Geometry check sheet. Reference: the model listing, model coordinates, mm. Face numbers are marked on the shaded views. A direction names the side the tool comes from. Give positions to 0.01 mm unless a question says otherwise; leave off trailing zeros. Loops run counter-clockwise (first coordinate to the right, second up) from the corner with the lowest first, then second, coordinate; pieces in that order, holes last. Notation, with made-up numbers: (66, 22.25) -> (103, 22.25) arc R25 ccw to (103, 58.25) -> close; hole circle Ø1 at (83.25, -34.75). An arc over 180 degrees is marked (long way). Answer in a Markdown table with one row per item. Add a question column.
Autodesk Inventor part; units mm, degrees
ref_plane "YZ Plane" through (0, 0, 0) normal (1, 0, 0) x (0, 1, 0)
ref_plane "XZ Plane" through (0, 0, 0) normal (0, 1, 0) x (-1, 0, 0)
ref_plane "XY Plane" through (0, 0, 0) normal (0, 0, 1) x (1, 0, 0)
sketch "Sketch1" plane through (0, 0, 0) normal (0, 1, 0) x (-1, 0, 0)
  line L0 (0, 0) -> (203.2, 0)
  line L1 (203.2, 0) -> (203.2, 25.4)
  line L2 (203.2, 25.4) -> (0, 25.4) construction
  line L3 (0, 25.4) -> (0, 0)
  line L4 (11.45, 12.7) -> (77.45, 12.7) construction
  circle A0 centre (11.45, 12.7) radius 3.302
  circle A1 centre (77.45, 12.7) radius 3.302
  line L5 (44.45, 25.4) -> (44.45, 0) construction
  circle A2 centre (127, 12.7) radius 3.302
  circle A3 centre (177.8, 12.7) radius 3.302
  line L6 (127, 12.7) -> (177.8, 12.7) construction
  line L7 (152.4, 25.4) -> (152.4, 0) construction
  line L8 (0, 25.4) -> (0, 101.6)
  line L9 (0, 101.6) -> (203.2, 101.6)
  line L10 (203.2, 101.6) -> (203.2, 25.4)
  point P0 (44.45, 12.7)
  point P1 (152.4, 12.7)
  dimension "d0" = 66
  dimension "d1" = 6.604
  dimension "d2" = 6.604
  dimension "d3" = 25.4
  dimension "d4" = 44.45
  dimension "d6" = 50.8
  dimension "d7" = 50.8
  dimension "d8" = 76.2
  dimension "d9" = 203.2
extrude "Plate1" add sketch "Sketch1" along normal blind 3.175
sketch "Sketch2" plane through (-203.2, 3.175, 98.425) normal (0, 0, 1) x (1, 0, 0)
  line L0 (203.2, 0) -> (0, 0)
  line L1 (0, 0) -> (0, -50.8)
  line L2 (0, -50.8) -> (203.2, -50.8)
  line L3 (203.2, -50.8) -> (203.2, 0)
edge flange "Flange1" height 50.8 angle 90 thickness 3.175 bend radius 1.27 thickness toward (0, 0, 1) relief tear relief width 3.175 relief depth 1.5875 edges at (-101.6, 0, 101.6) wall of the first edge with corners at (0, 3.175, 98.425) (-203.2, 3.175, 98.425) (-203.2, -47.625, 98.425) (0, -47.625, 98.425)
bend "Bend1"
corner "Corner1"
equation "\"d11\" = BendReliefWidth"
equation "\"d12\" = BendReliefDepth"
equation "\"d13\" = MinimumRemnant"
equation "\"d14\" = BendRadius"
equation "\"d18\" = CornerReliefSize"
equation "\"d19\" = GapSize"
equation "\"d20\" = JacobiRadiusSize"
equation "\"BendRadius\" = Thickness"
equation "\"BendReliefWidth\" = Thickness"
equation "\"BendReliefDepth\" = 0.5 * Thickness"
equation "\"CornerReliefSize\" = 4 * Thickness"
equation "\"MinimumRemnant\" = 2 * Thickness"
equation "\"TransitionRadius\" = BendRadius"
equation "\"JacobiRadiusSize\" = BendRadius"
equation "\"GapSize\" = Thickness"
equation "\"d10\" = BendRadius"
properties part number "Electrical Board Mount Part1" material "Aluminum 6061"
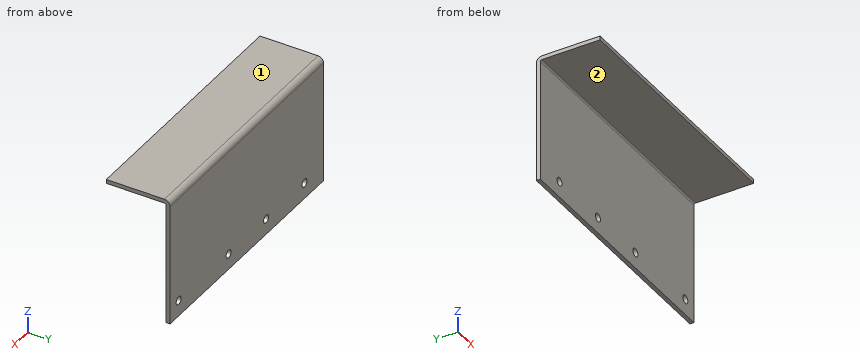
1. Sectioned sample at D-D (y = -44). Enter the section's corners in (x, z) (3 decimals).
2. Sectioned sample at B-B (x = -47). Enter the section's corners in (y, z) (3 decimals), plus the area to 3 significant figures.
3. Access from +Z, -Z, +X, -X, +Y, -Y to the whole of each face (thin tool, end or side, straight path). Record for the marked faces 1 and 2.
4. Gauge pin test, flat ends, axial feed: pin 1 Ø10.5 at (x, z) = (-127, 12.7) entering from -Y; pin 2 Ø4 at (x, y) = (-105, -13) entering from -Z (3 decimals). Record the tip position at first contact, or that the pin passes through.
5. Sectioned sample at C-C (z = 39). Enter the section's corners in (x, y) (3 decimals), plus the area to 3 significant figures.
6. Sectioned sample at A-A (x = -77.45). Enter the section's corners in (y, z) (3 decimals).
7. Material ranges on L1, parallel to Y at x = -111, z = 73 (3 decimals); L2, parallel to Z at x = -77.45, y = 0.7; L3, parallel to Z at x = -65, y = -21 (3 decimals), recorded low to high. Write a range as from..to.
Response:
| question | item | result |
|---|---|---|
| 1 | outline | (-203.2, 98.425) -> (0, 98.425) -> (0, 101.6) -> (-203.2, 101.6) -> close |
| 2 | outline | (-47.625, 98.425) -> (-1.27, 98.425) arc R1.27 cw to (0, 97.155) -> (0, 0) -> (3.175, 0) -> (3.175, 97.155) arc R4.445 ccw to (-1.27, 101.6) -> (-47.625, 101.6) -> close |
| 2 | area | 470 mm2 |
| 3 | face 1 | +Z, +X, -X, +Y, -Y |
| 3 | face 2 | -Z, +X, -X, -Y |
| 4 | pin 1 | stops at y = 0 |
| 4 | pin 2 | stops at z = 98.425 |
| 5 | outline | (-203.2, 0) -> (0, 0) -> (0, 3.175) -> (-203.2, 3.175) -> close |
| 5 | area | 645 mm2 |
| 6 | outline | (-47.625, 98.425) -> (-1.27, 98.425) arc R1.27 cw to (0, 97.155) -> (0, 16.002) -> (3.175, 16.002) -> (3.175, 97.155) arc R4.445 ccw to (-1.27, 101.6) -> (-47.625, 101.6) -> close; (0, 0) -> (3.175, 0) -> (3.175, 9.398) -> (0, 9.398) -> close |
| 7 | L1 | y = 0..3.175 |
| 7 | L2 | z = 0..9.4, 16..101.14 |
| 7 | L3 | z = 98.425..101.6 |
